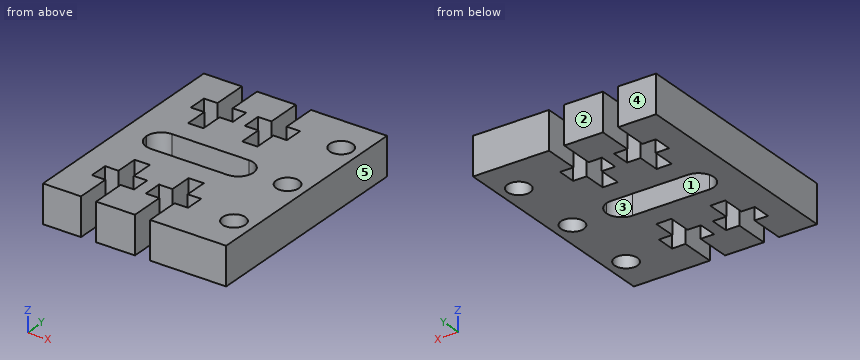
from build123d import *

# Parameters (mm, degrees)
ESBO_O1_W                = 24.096
ESBO_O1_H                = 30
RESSALTO_EXTRUS_O1_DEPTH = 5
ESBO_O2_R                = 1.5
CORTE_EXTRUS_O1_DEPTH    = 10
CORTE_EXTRUS_O2_DEPTH    = 6
CORTE_EXTRUS_O3_DEPTH    = 10
ESBO_O5_R                = 1.5
CORTE_EXTRUS_O4_DEPTH    = 6


with BuildPart() as part:
    # Esboço1 → Ressalto-extrusão1 (new body)
    with BuildSketch(Plane.XY):
        with Locations((-8.476916648, -30.459463918)):
            Rectangle(ESBO_O1_W, ESBO_O1_H)
    extrude(amount=RESSALTO_EXTRUS_O1_DEPTH)

    # Esboço2 → Corte-extrusão1 (cut)
    with BuildSketch(Plane(origin=(0, 0, 0), x_dir=(-1, 0, 0), z_dir=(0, 0, -1))):
        with Locations((-1.071083352, -30.459463918)):
            Circle(ESBO_O2_R)
        with Locations((-1.071083352, -20.459463918)):
            Circle(ESBO_O2_R)
    extrude(amount=-CORTE_EXTRUS_O1_DEPTH, mode=Mode.SUBTRACT)

    # Esboço3 → Corte-extrusão2 (cut, through all)
    with BuildSketch(Plane(origin=(0, 0, 0), x_dir=(-1, 0, 0), z_dir=(0, 0, -1))):
        Polygon((15.524916648, -15.459463918), (13.524916648, -15.459463918), (13.524916648, -20.009463918), (11.754916648, -20.009463918), (11.754916648, -22.459463918), (13.524916648, -22.459463918), (13.524916648, -25.459463918), (15.524916648, -25.459463918), (15.524916648, -22.459463918), (17.294916648, -22.459463918), (17.294916648, -20.009463918), (15.524916648, -20.009463918), align=None)
        Polygon((8.428916648, -15.459463918), (6.428916648, -15.459463918), (6.428916648, -20.009463918), (4.658916648, -20.009463918), (4.658916648, -22.459463918), (6.428916648, -22.459463918), (6.428916648, -25.459463918), (8.428916648, -25.459463918), (8.428916648, -22.459463918), (10.198916648, -22.459463918), (10.198916648, -20.009463918), (8.428916648, -20.009463918), align=None)
        Polygon((6.428916648, -40.909463918), (4.658916648, -40.909463918), (4.658916648, -38.459463918), (6.428916648, -38.459463918), (6.428916648, -35.459463918), (8.428916648, -35.459463918), (8.428916648, -38.459463918), (10.198916648, -38.459463918), (10.198916648, -40.909463918), (8.428916648, -40.909463918), (8.428916648, -45.459463918), (6.428916648, -45.459463918), align=None)
        Polygon((13.524916648, -40.909463918), (11.754916648, -40.909463918), (11.754916648, -38.459463918), (13.524916648, -38.459463918), (13.524916648, -35.459463918), (15.524916648, -35.459463918), (15.524916648, -38.459463918), (17.294916648, -38.459463918), (17.294916648, -40.909463918), (15.524916648, -40.909463918), (15.524916648, -45.459463918), (13.524916648, -45.459463918), align=None)
    extrude(amount=-CORTE_EXTRUS_O2_DEPTH, mode=Mode.SUBTRACT)

    # Esboço4 → Corte-extrusão3 (cut)
    with BuildSketch(Plane(origin=(0, 0, 0), x_dir=(-1, 0, 0), z_dir=(0, 0, -1))):
        with BuildLine():
            Line((15.534916648, -32.459463918), (5.415284958, -32.459463918))
            ThreePointArc((5.415284958, -32.459463918), (4.008142463, -31.876606412), (3.425284958, -30.469463918))
            Line((3.425284958, -30.469463918), (3.425284958, -30.449463918))
            ThreePointArc((3.425284958, -30.449463918), (4.008142463, -29.042321423), (5.415284958, -28.459463918))
            Line((5.415284958, -28.459463918), (15.534916648, -28.459463918))
            ThreePointArc((15.534916648, -28.459463918), (16.942059143, -29.042321423), (17.524916648, -30.449463918))
            Line((17.524916648, -30.449463918), (17.524916648, -30.469463918))
            ThreePointArc((17.524916648, -30.469463918), (16.942059143, -31.876606412), (15.534916648, -32.459463918))
        make_face()
    extrude(amount=-CORTE_EXTRUS_O3_DEPTH, mode=Mode.SUBTRACT)

    # Esboço5 → Corte-extrusão4 (cut, through all)
    with BuildSketch(Plane.XY.offset(5)):
        with Locations((1.071083352, -40.459463918)):
            Circle(ESBO_O5_R)
    extrude(amount=-CORTE_EXTRUS_O4_DEPTH, mode=Mode.SUBTRACT)


solid = part.part
Design review of the part built by this model. Coordinates are the model's own, in mm. Face numbers are marked on the shaded views. A direction names the side the tool comes from. Coordinates: 2 decimals unless noted, no trailing zeros. Loops run counter-clockwise (first coordinate to the right, second up) from the corner with the lowest first, then second, coordinate; pieces in that order, holes last. Notation, with made-up numbers: (55, 82) -> (114, 82) arc R14 ccw to (114, 100) -> close; hole circle Ø1 at (31.25, 31). An arc over 180 degrees is marked (long way). Use a Markdown table: item, result. Add a question column.
Item 1: Clearance check with a flat-ended pin moving along its axis: P1, Ø2, axis at x = -7.5, z = 2, coming from the +Y side. State where the tip first meets the part, or that it passes through.
Item 2: We need section C-C, the plane x = 1.25. Write out the cut boundary in (y, z).
Item 3: Machinability: for the marked faces 1 and 2, which of the approach directions +Z, -Z, +X, -X, +Y, -Y give a long, thin tool a straight path to every point of the face, cutting with its end or side? Answer none if there is none.
Item 4: Wall thickness on L1, parallel to X at y = -25, z = 1.9; L2, parallel to Y at x = -12.5, z = 4.5; L3, parallel to X at y = -40.5, z = 1.3: over which ranges is each line inside the solid? List them lowest first. Write a range as from..to.
Item 5: The part is to be moulded in two halves that separate along Y. For the marked faces 3, 4 and 5, say which applies: +Y half, -Y half, draft (parallel to the pull), parting line (faces both ways), or undercut.
Item 6: We need section D-D, the plane z = 1. Count the separate pieces of the cut face and the enclosed holes in it, and give its area (3 significant figures).
Item 7: We need section A-A, the plane y = -18.25. Write out the cut boundary in (x, z), and give its area (3 significant figures).
Item 8: We need section B-B, the plane x = -9. Write out the cut boundary in (y, z), and give its area (4 significant figures).
Numbers:
| question | item | result |
|---|---|---|
| 1 | P1 | stops at y = -15.46 |
| 2 | outline | (-45.46, 0) -> (-41.95, 0) -> (-41.95, 5) -> (-45.46, 5) -> close; (-38.97, 0) -> (-31.95, 0) -> (-31.95, 5) -> (-38.97, 5) -> close; (-28.97, 0) -> (-21.95, 0) -> (-21.95, 5) -> (-28.97, 5) -> close; (-18.97, 0) -> (-15.46, 0) -> (-15.46, 5) -> (-18.97, 5) -> close |
| 3 | face 1 | +Z, -Z |
| 3 | face 2 | +Z, -Z, +X, -X, +Y |
| 4 | L1 | x = -20.52..-15.52, -13.52..-8.43, -6.43..3.57 |
| 4 | L2 | y = -45.46..-40.91, -38.46..-32.46, -28.46..-22.46, -20.01..-15.46 |
| 4 | L3 | x = -20.52..-17.29, -11.75..-10.2, -4.66..-0.43, 2.57..3.57 |
| 5 | face 3 | undercut |
| 5 | face 4 | +Y half |
| 5 | face 5 | draft |
| 6 | separate pieces | 1 |
| 6 | enclosed holes | 4 |
| 6 | area | 534 mm^2 |
| 7 | outline | (-20.52, 0) -> (-15.52, 0) -> (-15.52, 5) -> (-20.52, 5) -> close; (-13.52, 0) -> (-8.43, 0) -> (-8.43, 5) -> (-13.52, 5) -> close; (-6.43, 0) -> (3.57, 0) -> (3.57, 5) -> (-6.43, 5) -> close |
| 7 | area | 100 mm^2 |
| 8 | outline | (-45.46, 0) -> (-40.91, 0) -> (-40.91, 5) -> (-45.46, 5) -> close; (-38.46, 0) -> (-32.46, 0) -> (-32.46, 5) -> (-38.46, 5) -> close; (-28.46, 0) -> (-22.46, 0) -> (-22.46, 5) -> (-28.46, 5) -> close; (-20.01, 0) -> (-15.46, 0) -> (-15.46, 5) -> (-20.01, 5) -> close |
| 8 | area | 105.5 mm^2 |
